Can you work these out from the model? Positions are in its coordinate system, mm. A direction names the side the tool comes from. Coordinates: 2 decimals unless noted, no trailing zeros. Loops run counter-clockwise (first coordinate to the right, second up) from the corner with the lowest first, then second, coordinate; pieces in that order, holes last. Notation, with made-up numbers: (-33.75, -14) - (-27.75, -14) arc R7 ccw to (-27.75, -9) - close; hole circle Ø3 at (79.5, 60). An arc over 180 degrees is marked (long way). Put each result on its own line as item: value. Start each with the question number.
from build123d import *

# Parameters (mm, degrees)
SKETCH11_R          = 288.5
SKETCH11_R_2        = 269.571318971
SKETCH11_W          = 21.16178464
SKETCH11_H          = 20.378014839
BOSS_EXTRUDE7_DEPTH = 10
SKETCH11_7_W        = 21.16178464
SKETCH11_7_H        = 20.378014839
BOSS_EXTRUDE8_DEPTH = 5
BOSS_EXTRUDE9_DEPTH = 15


with BuildPart() as part:
    # Sketch11 → Boss-Extrude7 (new body)
    # profile 1 of 6: a face of its own
    with BuildSketch(Plane.YZ):
        with Locations(Location((288.5, 288.5, 0), (0, 0, 270))):
            Circle(SKETCH11_R)
        with Locations((288.5, 288.5)):
            Circle(SKETCH11_R_2, mode=Mode.SUBTRACT)
    # profile 2 of 6: a face of its own
    with BuildSketch(Plane.YZ):
        with BuildLine():
            ThreePointArc((308.145483606, 557.354516394), (288.5, 558.071318971), (268.854516394, 557.354516394))
            Line((268.854516394, 557.354516394), (201.425647915, 489.925647915))
            Line((201.425647915, 489.925647915), (109.345306024, 489.925647915))
            ThreePointArc((109.345306024, 489.925647915), (98.277565899, 479.508171491), (87.814555723, 468.483467205))
            Line((87.814555723, 468.483467205), (87.814555723, 376.314555723))
            Line((87.814555723, 376.314555723), (19.645483606, 308.145483606))
            ThreePointArc((19.645483606, 308.145483606), (18.928681029, 288.5), (19.645483606, 268.854516394))
            Line((19.645483606, 268.854516394), (87.814555723, 200.685444277))
            Line((87.814555723, 200.685444277), (87.814555723, 108.516532795))
            ThreePointArc((87.814555723, 108.516532795), (97.646860109, 98.122020693), (108.016830289, 88.263835777))
            Line((108.016830289, 88.263835777), (200.236164223, 88.263835777))
            Line((200.236164223, 88.263835777), (268.854516394, 19.645483606))
            ThreePointArc((268.854516394, 19.645483606), (288.5, 18.928681029), (308.145483606, 19.645483606))
            Line((308.145483606, 19.645483606), (376.763835777, 88.263835777))
            Line((376.763835777, 88.263835777), (468.983169711, 88.263835777))
            ThreePointArc((468.983169711, 88.263835777), (479.697404879, 98.467770157), (489.835656115, 109.244178369))
            Line((489.835656115, 109.244178369), (489.835656115, 201.335656115))
            Line((489.835656115, 201.335656115), (557.354516394, 268.854516394))
            ThreePointArc((557.354516394, 268.854516394), (557.892058724, 278.670721898), (558.071318971, 288.5))
            ThreePointArc((558.071318971, 288.5), (557.892058724, 298.329278102), (557.354516394, 308.145483606))
            Line((557.354516394, 308.145483606), (489.835656115, 375.664343885))
            Line((489.835656115, 375.664343885), (489.835656115, 467.755821631))
            ThreePointArc((489.835656115, 467.755821631), (479.067840748, 479.16356255), (467.654693976, 489.925647915))
            Line((467.654693976, 489.925647915), (375.574352085, 489.925647915))
            Line((375.574352085, 489.925647915), (308.145483606, 557.354516394))
        make_face()
        Polygon((118.728003632, 357.153372391), (118.728003632, 456.354802066), (217.929433307, 456.354802066), (288.5, 526.925368759), (359.070566693, 456.354802066), (457.657670049, 456.354802066), (457.657670049, 357.76769871), (525.597184912, 289.828183847), (457.657670049, 221.888668984), (457.657670049, 119.01635474), (359.070566693, 119.01635474), (354.785355806, 119.01635474), (287.171816153, 51.402815088), (219.558276501, 119.01635474), (217.219769177, 119.01635474), (118.728003632, 119.01635474), (118.728003632, 219.846627609), (50.074631241, 288.5), align=None, mode=Mode.SUBTRACT)
    # profile 3 of 6: a face of its own
    with BuildSketch(Plane.YZ):
        Polygon((125.489898595, 388.458487724), (125.489898595, 450.488919168), (201.425647915, 450.488919168), (201.425647915, 349.632569577), (125.489898595, 349.632569577), (125.489898595, 370.245546136), (182.175584131, 370.245546136), (182.175584131, 388.458487724), align=None)
    # profile 4 of 6: a face of its own
    with BuildSketch(Plane.YZ):
        Polygon((232.103371973, 450.488919168), (232.103371973, 369.045528651), (206.163784466, 370.245546136), (206.163784466, 349.632569577), (252.593459139, 349.632569577), (252.593459139, 388.458487724), (322.412082429, 388.458487724), (322.412082429, 349.632569577), (452.588861428, 349.632569577), (452.588861428, 450.488919168), (375.574352085, 450.488919168), (375.574352085, 369.045528651), (343.349626731, 369.045528651), (343.349626731, 450.488919168), (322.412082429, 450.488919168), (322.412082429, 409.767223909), (252.593459139, 409.767223909), (252.593459139, 450.488919168), align=None)
    # profile 5 of 6: a face of its own
    with BuildSketch(Plane.YZ):
        with Locations((308.504184867, 465.124823328)):
            Rectangle(SKETCH11_W, SKETCH11_H)
    # profile 6 of 6: a face of its own
    with BuildSketch(Plane.YZ):
        with Locations((269.315694793, 465.124823328)):
            Rectangle(SKETCH11_W, SKETCH11_H)
    extrude(amount=BOSS_EXTRUDE7_DEPTH)

    # Sketch11_7 → Boss-Extrude8 (add)
    # profile 1 of 10: a face of its own
    with BuildSketch(Plane.YZ):
        with BuildLine():
            Line((201.425647915, 489.925647915), (268.854516394, 557.354516394))
            ThreePointArc((268.854516394, 557.354516394), (183.537908139, 536.797513648), (109.345306024, 489.925647915))
            Line((109.345306024, 489.925647915), (201.425647915, 489.925647915))
        make_face()
    # profile 2 of 10: a face of its own
    with BuildSketch(Plane.YZ):
        with BuildLine():
            ThreePointArc((467.654693976, 489.925647915), (393.462091861, 536.797513648), (308.145483606, 557.354516394))
            Line((308.145483606, 557.354516394), (375.574352085, 489.925647915))
            Line((375.574352085, 489.925647915), (467.654693976, 489.925647915))
        make_face()
    # profile 3 of 10: a face of its own
    with BuildSketch(Plane.YZ):
        with BuildLine():
            Line((87.814555723, 376.314555723), (87.814555723, 468.483467205))
            ThreePointArc((87.814555723, 468.483467205), (40.419345952, 393.973622763), (19.645483606, 308.145483606))
            Line((19.645483606, 308.145483606), (87.814555723, 376.314555723))
        make_face()
    # profile 4 of 10: a face of its own
    with BuildSketch(Plane.YZ):
        with BuildLine():
            ThreePointArc((557.354516394, 308.145483606), (536.771151329, 393.524432536), (489.835656115, 467.755821631))
            Line((489.835656115, 467.755821631), (489.835656115, 375.664343885))
            Line((489.835656115, 375.664343885), (557.354516394, 308.145483606))
        make_face()
    # profile 5 of 10: a face of its own
    with BuildSketch(Plane.YZ):
        with BuildLine():
            Line((87.814555723, 200.685444277), (19.645483606, 268.854516394))
            ThreePointArc((19.645483606, 268.854516394), (40.419345952, 183.026377237), (87.814555723, 108.516532795))
            Line((87.814555723, 108.516532795), (87.814555723, 200.685444277))
        make_face()
    # profile 6 of 10: a face of its own
    with BuildSketch(Plane.YZ):
        with BuildLine():
            ThreePointArc((489.835656115, 109.244178369), (536.771151329, 183.475567464), (557.354516394, 268.854516394))
            Line((557.354516394, 268.854516394), (489.835656115, 201.335656115))
            Line((489.835656115, 201.335656115), (489.835656115, 109.244178369))
        make_face()
    # profile 7 of 10: a face of its own
    with BuildSketch(Plane.YZ):
        with BuildLine():
            Line((200.236164223, 88.263835777), (108.016830289, 88.263835777))
            ThreePointArc((108.016830289, 88.263835777), (182.717255503, 40.550999239), (268.854516394, 19.645483606))
            Line((268.854516394, 19.645483606), (200.236164223, 88.263835777))
        make_face()
    # profile 8 of 10: a face of its own
    with BuildSketch(Plane.YZ):
        with BuildLine():
            ThreePointArc((308.145483606, 19.645483606), (394.282744497, 40.550999239), (468.983169711, 88.263835777))
            Line((468.983169711, 88.263835777), (376.763835777, 88.263835777))
            Line((376.763835777, 88.263835777), (308.145483606, 19.645483606))
        make_face()
    # profile 9 of 10: a face of its own
    with BuildSketch(Plane.YZ):
        Polygon((217.929433307, 456.354802066), (118.728003632, 456.354802066), (118.728003632, 357.153372391), (50.074631241, 288.5), (118.728003632, 219.846627609), (118.728003632, 342.490695719), (219.558276501, 342.490695719), (288.5, 273.54897222), (359.070566693, 344.119538913), (457.657670049, 344.119538913), (457.657670049, 221.888668984), (525.597184912, 289.828183847), (457.657670049, 357.76769871), (457.657670049, 456.354802066), (359.070566693, 456.354802066), (288.5, 526.925368759), align=None)
        Polygon((125.489898595, 388.458487724), (125.489898595, 450.488919168), (201.425647915, 450.488919168), (201.425647915, 349.632569577), (125.489898595, 349.632569577), (125.489898595, 370.245546136), (182.175584131, 370.245546136), (182.175584131, 388.458487724), align=None, mode=Mode.SUBTRACT)
        with Locations((269.315694793, 465.124823328)):
            Rectangle(SKETCH11_7_W, SKETCH11_7_H, mode=Mode.SUBTRACT)
        Polygon((206.163784466, 349.632569577), (206.163784466, 370.245546136), (232.103371973, 369.045528651), (232.103371973, 450.488919168), (252.593459139, 450.488919168), (252.593459139, 409.767223909), (322.412082429, 409.767223909), (322.412082429, 450.488919168), (343.349626731, 450.488919168), (343.349626731, 369.045528651), (375.574352085, 369.045528651), (375.574352085, 450.488919168), (452.588861428, 450.488919168), (452.588861428, 349.632569577), (322.412082429, 349.632569577), (322.412082429, 388.458487724), (252.593459139, 388.458487724), (252.593459139, 349.632569577), align=None, mode=Mode.SUBTRACT)
        with Locations((308.504184867, 465.124823328)):
            Rectangle(SKETCH11_7_W, SKETCH11_7_H, mode=Mode.SUBTRACT)
    # profile 10 of 10: a face of its own
    with BuildSketch(Plane.YZ):
        Polygon((217.219769177, 197.201333657), (217.219769177, 119.01635474), (219.558276501, 119.01635474), (287.171816153, 51.402815088), (354.785355806, 119.01635474), (359.070566693, 119.01635474), (359.070566693, 201.335656115), (286.078006706, 128.343096128), align=None)
    extrude(amount=BOSS_EXTRUDE8_DEPTH)

    # Sketch11_8 → Boss-Extrude9 (add)
    with BuildSketch(Plane.YZ):
        Polygon((118.728003632, 342.490695719), (118.728003632, 219.846627609), (118.728003632, 119.01635474), (217.219769177, 119.01635474), (217.219769177, 197.201333657), (286.078006706, 128.343096128), (359.070566693, 201.335656115), (359.070566693, 119.01635474), (457.657670049, 119.01635474), (457.657670049, 221.888668984), (457.657670049, 344.119538913), (359.070566693, 344.119538913), (288.5, 273.54897222), (219.558276501, 342.490695719), align=None)
    extrude(amount=BOSS_EXTRUDE9_DEPTH)


solid = part.part
Q1. Please list where these lines run through material, in increasing order: line 1 along Z through (x, y) = (6, 529); line 2 along Z through (x, y) = (5.5, 389); line 3 along Y through (x, z) = (7.5, 216). Write a range as [from, to].
Q2. I want a section at A-A on x = 7.75. Count the separate pieces of the cut face and the enclosed holes in it, and give its area (3 significant figures).
Q3. Will these pins go through, and if not, where does the flat tip stop? pin 1 (4 mm diameter, centred on x = 12.5, y = 428.5, fed in from -Z); pin 2 (5.5 mm diameter, centred on x = 8, z = 434.5, fed in from -Y); pin 3 (5.5 mm diameter, centred on x = 7, y = 159.5, fed in from +Z); pin 4 (3 mm diameter, centred on x = 12, z = 491, fed in from -Y).
Q4. On a 3-axis mill with a long thin cutter (end or side, diameter ignored), from which of +Z, -Z, +X, -X, +Y, -Y can I reach the whole of each face in a straight line? I mean faces 1 (the flat face through (10, 328, 401)), 2 (the flat face through (7.5, 342.3, 523.2)). Say none if no direction works.
Q5. I want a section at D-D on z = 144. List the corners of the cut face in (x, y) for me, and give its area (3 significant figures).
Q6. We'd pull the mould along X, two halves only. Please class faces 3 (the flat face through (5, 61, 389)), 4 (the flat face through (9.93, 322.063, 164.328)): released by +X, released by -X, zero draft, split by the parting line, or undercut.
Q7. I want a section at B-B on z = 518.5. List the corners of the cut face in (x, y) for me, and give its area (3 significant figures).
Calculated:
1. line 1: [129.15, 166.73], [240.5, 336.5], [410.27, 447.85]
1. line 2: [18.07, 38.36], [88.26, 344.12], [349.63, 450.49], [456.35, 489.93], [538.64, 558.93]
1. line 3: [9.26, 28.86], [72.5, 504.5], [548.14, 567.74]
2. separate pieces: 5
2. enclosed holes: 10
2. area: 177,000 mm2
3. pin 1: z = 119.02
3. pin 2: y = 38.08
3. pin 3: z = 547.91
3. pin 4: through
4. face 1: +Z, +X, +Y, -Y
4. face 2: +X
5. outline: (0, 38.8) - (10, 38.8) - (10, 60.93) - (5, 60.93) - (5, 87.81) - (10, 87.81) - (10, 118.73) - (15, 118.73) - (15, 217.22) - (5, 217.22) - (5, 270.42) - (15, 270.42) - (15, 301.73) - (5, 301.73) - (5, 359.07) - (15, 359.07) - (15, 457.66) - (10, 457.66) - (10, 489.84) - (5, 489.84) - (5, 516.07) - (10, 516.07) - (10, 538.2) - (0, 538.2) - close
5. area: 5,320 mm2
6. face 3: released by +X
6. face 4: zero draft
7. outline: (0, 114.34) - (10, 114.34) - (10, 147.9) - (5, 147.9) - (5, 230) - (10, 230) - (10, 280.07) - (5, 280.07) - (5, 296.93) - (10, 296.93) - (10, 347) - (5, 347) - (5, 429.1) - (10, 429.1) - (10, 462.66) - (0, 462.66) - close
7. area: 2,580 mm2
